Verification items for this drawing (mm, ordinates from the low corner). A direction names the side the tool comes from. Give positions to 0.01 mm unless a question says otherwise; leave off trailing zeros. Write each loop counter-clockwise with the first axis right and the second up, starting at its lowest first coordinate (ties: lowest second). Pieces come first, ordered by that corner, then holes. Notation, with made-up numbers: (15, 51.25) -> (40, 51.25) arc R19 cw to (40, 63.25) -> close; hole circle Ø7 at (89.5, 88.25). An arc over 180 degrees is marked (long way). Use one line per item in the form item = value. Start each with the question number.
(1) Section check C-C, the plane y = 6. Record the cut outline in (x, z).
(2) Section check B-B, the plane x = 25.5. Record the cut outline in (y, z).
(3) Scan lines: L1, parallel to Y at x = 11.5, z = 17.5; L2, parallel to X at y = 32, z = 26.5; L3, parallel to Z at x = 8.5, y = 20.5. Record each from-to range of solid material in increasing order.
(4) Set-up check for the marked faces 1 and 2: record each of +Z, -Z, +X, -X, +Y, -Y from which the full face is reachable in a straight line by a thin tool's end or side.
(5) Depth check by flat-ended pin: pin 1 Ø12.5 at (x, y) = (15.5, 16.5) entering from -Z; pin 2 Ø7.5 at (y, z) = (21, 12) entering from +X; pin 3 Ø5 at (x, z) = (20.5, 20) entering from -Y; pin 4 Ø4 at (y, z) = (8.5, 30) entering from +X. Enter the tip coordinate at first touch or a pass-through.
(6) Section check D-D, the plane y = 19.5. Record the cut outline in (x, z).
(7) Section check A-A, the plane z = 7.5. Record the cut outline in (x, y).
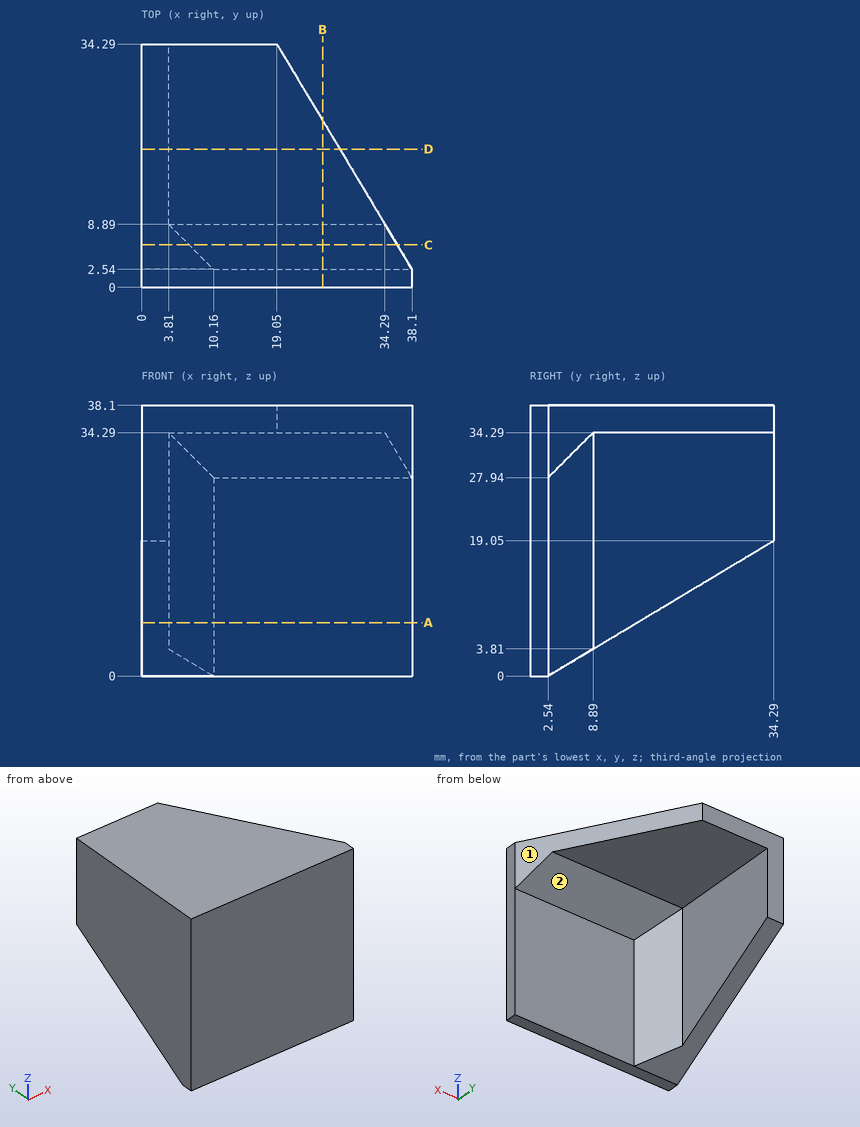
Completed:
q1.outline = (0, 2.08) -> (6.7, 2.08) -> (6.7, 31.4) -> (36.02, 31.4) -> (36.02, 38.1) -> (0, 38.1) -> close
q2.outline = (0, 0) -> (2.54, 0) -> (2.54, 27.94) -> (8.89, 34.29) -> (23.54, 34.29) -> (23.54, 38.1) -> (0, 38.1) -> close
q3.L1 = 0 to 2.54
q3.L2 = 0 to 3.81
q3.L3 = 34.29 to 38.1
q4.face_1 = +Z, -Z, +X, +Y
q4.face_2 = -Z, +X, +Y
q5.pin_1 = 34.29
q5.pin_2 = 3.81
q5.pin_3 = 0
q5.pin_4 = 6.2
q6.outline = (0, 10.18) -> (3.81, 10.18) -> (3.81, 34.29) -> (27.92, 34.29) -> (27.92, 38.1) -> (0, 38.1) -> close
q7.outline = (0, 0) -> (38.1, 0) -> (38.1, 2.54) -> (10.16, 2.54) -> (3.81, 8.89) -> (3.81, 15.04) -> (0, 15.04) -> close
